from build123d import *

# Parameters (mm, degrees)
SKETCH2_R               = 3
BOSS_EXTRUDE1_DEPTH     = 15
SKETCH3_W               = 4
SKETCH3_H               = 5.183202584
CUT_EXTRUDE1_DEPTH      = 7
CUT_EXTRUDE4_DEPTH      = 6
CUT_EXTRUDE4_DEPTH_BACK = 3
SKETCH4_R               = 0.75
SKETCH12_R              = 2.5
BOSS_EXTRUDE2_DEPTH     = 1
SKETCH13_R              = 3
BOSS_EXTRUDE3_DEPTH     = 1.5
SKETCH14_R              = 2.5
BOSS_EXTRUDE4_DEPTH     = 1
SKETCH15_R              = 3
BOSS_EXTRUDE5_DEPTH     = 1.5
SKETCH16_R              = 2.5
BOSS_EXTRUDE6_DEPTH     = 1
SKETCH17_R              = 3
BOSS_EXTRUDE7_DEPTH     = 1.5
SKETCH18_R              = 2.5
BOSS_EXTRUDE8_DEPTH     = 1
SKETCH19_R              = 3
BOSS_EXTRUDE9_DEPTH     = 16.5
SKETCH28_R              = 2.5
BOSS_EXTRUDE11_DEPTH    = 80
FILLET6_R               = 2


with BuildPart() as part:
    # Sketch2 → Boss-Extrude1 (new body)
    with BuildSketch(Plane.XY):
        Circle(SKETCH2_R)
    extrude(amount=BOSS_EXTRUDE1_DEPTH)

    # Sketch3 → Cut-Extrude1 (cut)
    with BuildSketch(Plane(origin=(0, 0, 0), x_dir=(-1, 0, 0), z_dir=(0, 0, -1))):
        with Locations((0, 0.591601292)):
            Rectangle(SKETCH3_W, SKETCH3_H)
    extrude(amount=-CUT_EXTRUDE1_DEPTH, mode=Mode.SUBTRACT)

    # Sketch4 → Cut-Extrude4 (cut, two sides: drawn at the far end of the back side and taken through both)
    with BuildSketch(Plane(origin=(-2, 0, 0), x_dir=(0, 0, -1), z_dir=(1, 0, 0)).offset(-CUT_EXTRUDE4_DEPTH_BACK)):
        with Locations((-3.5, 0.236067977)):
            Circle(SKETCH4_R)
    extrude(amount=CUT_EXTRUDE4_DEPTH + CUT_EXTRUDE4_DEPTH_BACK, mode=Mode.SUBTRACT)

    # Sketch12 → Boss-Extrude2 (add)
    with BuildSketch(Plane.XY.offset(15)):
        Circle(SKETCH12_R)
    extrude(amount=BOSS_EXTRUDE2_DEPTH)

    # Sketch13 → Boss-Extrude3 (add)
    with BuildSketch(Plane.XY.offset(16)):
        with Locations(Location((0, 0, 0), (0, 0, 131.810314896))):
            Circle(SKETCH13_R)
    extrude(amount=BOSS_EXTRUDE3_DEPTH)

    # Sketch14 → Boss-Extrude4 (add)
    with BuildSketch(Plane.XY.offset(17.5)):
        Circle(SKETCH14_R)
    extrude(amount=BOSS_EXTRUDE4_DEPTH)

    # Sketch15 → Boss-Extrude5 (add)
    with BuildSketch(Plane.XY.offset(18.5)):
        with Locations(Location((0, 0, 0), (0, 0, 131.810314896))):
            Circle(SKETCH15_R)
    extrude(amount=BOSS_EXTRUDE5_DEPTH)

    # Sketch16 → Boss-Extrude6 (add)
    with BuildSketch(Plane.XY.offset(20)):
        Circle(SKETCH16_R)
    extrude(amount=BOSS_EXTRUDE6_DEPTH)

    # Sketch17 → Boss-Extrude7 (add)
    with BuildSketch(Plane.XY.offset(21)):
        with Locations(Location((0, 0, 0), (0, 0, 131.810314896))):
            Circle(SKETCH17_R)
    extrude(amount=BOSS_EXTRUDE7_DEPTH)

    # Sketch18 → Boss-Extrude8 (add)
    with BuildSketch(Plane.XY.offset(22.5)):
        Circle(SKETCH18_R)
    extrude(amount=BOSS_EXTRUDE8_DEPTH)

    # Sketch19 → Boss-Extrude9 (add)
    with BuildSketch(Plane.XY.offset(23.5)):
        with Locations(Location((0, 0, 0), (0, 0, 131.810314896))):
            Circle(SKETCH19_R)
    extrude(amount=BOSS_EXTRUDE9_DEPTH)

    # Sketch28 → Boss-Extrude11 (add)
    with BuildSketch(Plane.XY.offset(40)):
        Circle(SKETCH28_R)
    extrude(amount=BOSS_EXTRUDE11_DEPTH)

    # Fillet6
    fillet6_edges = [part.edges().sort_by_distance(p)[0] for p in [
        (-2.5, 0, 120),
    ]]
    fillet(fillet6_edges, radius=FILLET6_R)


solid = part.part
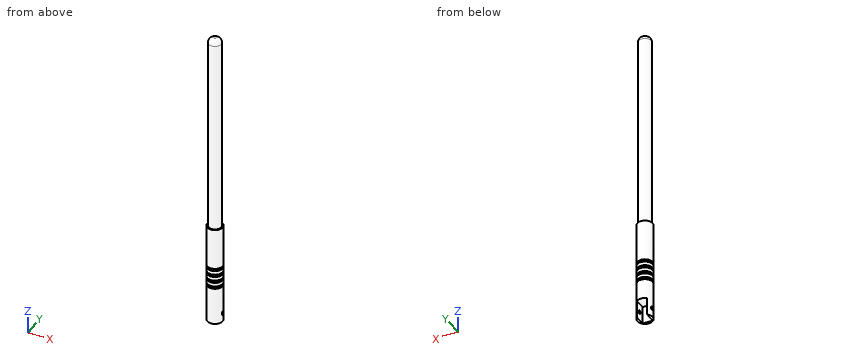
For this review, take the finished solid that the model builds, in its own axes (mm). Coordinates: 2 decimals unless noted, no trailing zeros. Write each loop counter-clockwise with the first axis right and the second up, starting at its lowest first coordinate (ties: lowest second). Pieces come first, ordered by that corner, then holes. Notation, with made-up numbers: (5, 68.5) -> (53, 68.5) arc R23 ccw to (53, 98.5) -> close; hole circle Ø5 at (40, -19.75). An arc over 180 degrees is marked (long way). Write each question's results on one line, items separated by ' | '. Start each with the question number.
1) Insertion check: pin 1 (1.5 mm diameter, centred on x = 1.5, z = 76.5, fed in from +Y); pin 2 (1 mm diameter, centred on y = -2, z = 99.5, fed in from +X); pin 3 (1.2 mm diameter, centred on x = -0.5, y = 1, fed in from -Z); pin 4 (3.5 mm diameter, centred on y = 1, z = 2.5, fed in from -X). Each pin has a flat end and moves straight along its axis. Give the tip position at first contact, or say it passes through.
2) Wall thickness on L1, parallel to Z at x = 2.5, y = -1; L2, parallel to Z at x = -0.5, y = 2.75; L3, parallel to Y at x = -2.6, z = 3.5: over which ranges is each line inside the solid? List them lowest first. Write a range as [from, to].
3) Consider section A-A (z = 112). Write out the cut boundary in (x, y).
Geometry says:
1) pin 1: y = 2.38 | pin 2: x = 2 | pin 3: z = 7 | pin 4: x = -3
2) L1: [0, 15], [16, 17.5], [18.5, 20], [21, 22.5], [23.5, 40] | L2: [7, 15], [16, 17.5], [18.5, 20], [21, 22.5], [23.5, 40] | L3: [-1.5, -0.51], [0.99, 1.5]
3) outline: circle Ø5 at (0, 0)
